Build history of the part. All positions in model axes, mm. Face numbers are marked on the shaded views. A direction names the side the tool comes from. Give positions to 0.01 mm unless a question says otherwise; leave off trailing zeros. Loops run counter-clockwise (first coordinate to the right, second up) from the corner with the lowest first, then second, coordinate; pieces in that order, holes last. Notation, with made-up numbers: (34.25, 16.5) -> (88.25, 16.5) arc R3 cw to (88.25, 20.5) -> close; hole circle Ø3 at (49, 49.5). An arc over 180 degrees is marked (long way). Answer in a Markdown table with one row per item. Add a question column.
from build123d import *

# Parameters (mm, degrees)
MAIN_BODY_DEPTH  = 77
LENS_CUT_DEPTH   = 3.1
END_RECESS_START = -77
END_RECESS_DEPTH = 1.05


with BuildPart() as part:
    # main_features_sketch → main_body (new, symmetric)
    with BuildSketch(Plane.XY):
        with BuildLine():
            ThreePointArc((24.721981093, -10.075200948), (21.063236898, -18.011630623), (12.946199947, -21.25))
            Line((12.946199947, -21.25), (-12.946199947, -21.25))
            ThreePointArc((-12.946199947, -21.25), (-21.063236898, -18.011630623), (-24.721981093, -10.075200948))
            Line((-24.721981093, -10.075200948), (-25.25, 0))
            Line((-25.25, 0), (-24.45, 0))
            Line((-24.45, 0), (-24.45, 0.6))
            Line((-24.45, 0.6), (-25.25, 0.6))
            Line((-25.25, 0.6), (-24.719878978, 10.11408323))
            ThreePointArc((-24.719878978, 10.11408323), (-21.049103134, 18.025020906), (-12.946199947, 21.25))
            Line((-12.946199947, 21.25), (12.946199947, 21.25))
            ThreePointArc((12.946199947, 21.25), (21.049103134, 18.025020906), (24.719878978, 10.11408323))
            Line((24.719878978, 10.11408323), (25.25, 0.6))
            Line((25.25, 0.6), (24.45, 0.6))
            Line((24.45, 0.6), (24.45, 0))
            Line((24.45, 0), (25.25, 0))
            Line((25.25, 0), (24.721981093, -10.075200948))
        make_face()
        with BuildLine():
            ThreePointArc((-23.124173837, -9.991463418), (-19.961869577, -16.85103163), (-12.946199947, -19.65))
            Line((-12.946199947, -19.65), (12.946199947, -19.65))
            ThreePointArc((12.946199947, -19.65), (19.961869577, -16.85103163), (23.124173837, -9.991463418))
            Line((23.124173837, -9.991463418), (23.5639518, -1.6))
            Line((23.5639518, -1.6), (22.85, -1.6))
            Line((22.85, -1.6), (22.85, 2.2))
            Line((22.85, 2.2), (23.558366806, 2.2))
            Line((23.558366806, 2.2), (23.12235695, 10.025069924))
            ThreePointArc((23.12235695, 10.025069924), (19.949653565, 16.86260504), (12.946199947, 19.65))
            Line((12.946199947, 19.65), (-12.946199947, 19.65))
            ThreePointArc((-12.946199947, 19.65), (-19.949653565, 16.86260504), (-23.12235695, 10.025069924))
            Line((-23.12235695, 10.025069924), (-23.558366806, 2.2))
            Line((-23.558366806, 2.2), (-22.85, 2.2))
            Line((-22.85, 2.2), (-22.85, -1.6))
            Line((-22.85, -1.6), (-23.5639518, -1.6))
            Line((-23.5639518, -1.6), (-23.124173837, -9.991463418))
        make_face(mode=Mode.SUBTRACT)
        with BuildLine():
            Line((-23.5639518, -1.6), (-23.124173837, -9.991463418))
            ThreePointArc((-23.124173837, -9.991463418), (-19.961869577, -16.85103163), (-12.946199947, -19.65))
            Line((-12.946199947, -19.65), (12.946199947, -19.65))
            ThreePointArc((12.946199947, -19.65), (19.961869577, -16.85103163), (23.124173837, -9.991463418))
            Line((23.124173837, -9.991463418), (23.5639518, -1.6))
            Line((23.5639518, -1.6), (22.85, -1.6))
            Line((22.85, -1.6), (22.85, 2.2))
            Line((22.85, 2.2), (23.558366806, 2.2))
            Line((23.558366806, 2.2), (23.12235695, 10.025069924))
            ThreePointArc((23.12235695, 10.025069924), (19.949653565, 16.86260504), (12.946199947, 19.65))
            Line((12.946199947, 19.65), (-12.946199947, 19.65))
            ThreePointArc((-12.946199947, 19.65), (-19.949653565, 16.86260504), (-23.12235695, 10.025069924))
            Line((-23.12235695, 10.025069924), (-23.558366806, 2.2))
            Line((-23.558366806, 2.2), (-22.85, 2.2))
            Line((-22.85, 2.2), (-22.85, -1.6))
            Line((-22.85, -1.6), (-23.5639518, -1.6))
        make_face()
    extrude(amount=MAIN_BODY_DEPTH, both=True)

    # lens_sketch → lens_cut (cut)
    with BuildSketch(Plane(origin=(0, 21.25, 0), x_dir=(1, 0, 0), z_dir=(0, 1, 0))):
        with BuildLine():
            Line((9.085700376, 58.2), (-9.085700376, 58.2))
            ThreePointArc((-9.085700376, 58.2), (-14.310724248, 56.035724248), (-16.475, 50.810700376))
            Line((-16.475, 50.810700376), (-16.475, 5.389299624))
            ThreePointArc((-16.475, 5.389299624), (-14.310724248, 0.164275752), (-9.085700376, -2))
            Line((-9.085700376, -2), (9.085700376, -2))
            ThreePointArc((9.085700376, -2), (14.310724248, 0.164275752), (16.475, 5.389299624))
            Line((16.475, 5.389299624), (16.475, 50.810700376))
            ThreePointArc((16.475, 50.810700376), (14.310724248, 56.035724248), (9.085700376, 58.2))
        make_face()
    extrude(amount=-LENS_CUT_DEPTH, mode=Mode.SUBTRACT)

    # Sketch1<3> → end_recess (cut)
    with BuildSketch(Plane.XY.offset(END_RECESS_START)):
        with BuildLine():
            Line((-23.5639518, -1.6), (-23.124173837, -9.991463418))
            ThreePointArc((-23.124173837, -9.991463418), (-19.961869577, -16.85103163), (-12.946199947, -19.65))
            Line((-12.946199947, -19.65), (12.946199947, -19.65))
            ThreePointArc((12.946199947, -19.65), (19.961869577, -16.85103163), (23.124173837, -9.991463418))
            Line((23.124173837, -9.991463418), (23.5639518, -1.6))
            Line((23.5639518, -1.6), (22.85, -1.6))
            Line((22.85, -1.6), (22.85, 2.2))
            Line((22.85, 2.2), (23.558366806, 2.2))
            Line((23.558366806, 2.2), (23.12235695, 10.025069924))
            ThreePointArc((23.12235695, 10.025069924), (19.949653565, 16.86260504), (12.946199947, 19.65))
            Line((12.946199947, 19.65), (-12.946199947, 19.65))
            ThreePointArc((-12.946199947, 19.65), (-19.949653565, 16.86260504), (-23.12235695, 10.025069924))
            Line((-23.12235695, 10.025069924), (-23.558366806, 2.2))
            Line((-23.558366806, 2.2), (-22.85, 2.2))
            Line((-22.85, 2.2), (-22.85, -1.6))
            Line((-22.85, -1.6), (-23.5639518, -1.6))
        make_face()
    end_recess = extrude(amount=END_RECESS_DEPTH, mode=Mode.SUBTRACT)

    # end_recess_2: end_recess across plane
    add(end_recess.mirror(Plane.XY), mode=Mode.SUBTRACT)


solid = part.part
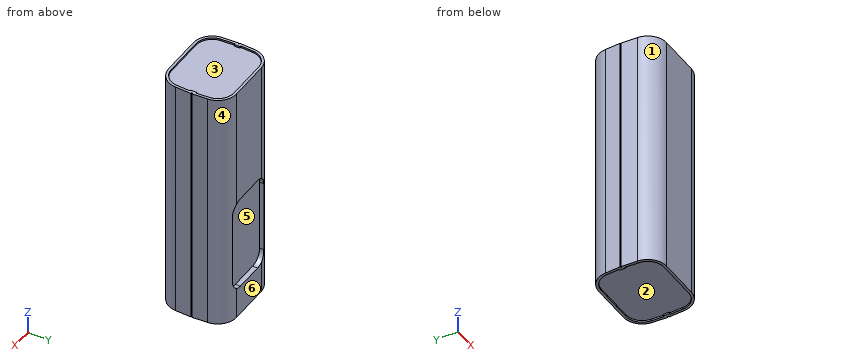
(1) 3-axis set-ups, long thin cutter, end or side, ignore diameter. For the marked faces 5 and 6: which of +Z, -Z, +X, -X, +Y, -Y reach the whole face in a straight line?
(2) Saw through at A-A, the plane z = -35. List the corners of the cut face in (x, y) (3 decimals).
(3) Flat gauge pins, fed straight in: pin 1 Ø4 at (y, z) = (13.5, -54) entering from -X; pin 2 Ø4 at (x, y) = (-17.5, 2.5) entering from +Z; pin 3 Ø12 at (x, y) = (7.5, -3.5) entering from -Z. Where does each tip first touch, or does it go through?
(4) Wall check: line 1 along Y through (x, z) = (3, -21.5); line 2 along Y through (x, z) = (13.5, 34); line 3 along Z through (x, y) = (-1.5, -8.5). Give the ranges that are in metal, low to high. Write a range as from..to.
(5) Saw through at D-D, the plane z = 66. List the corners of the cut face in (x, y).
(6) Two-plate mould, pull along Y, no slides. Class the marked faces 1, 2, 3 and 4: released by +Y, released by -Y, zero draft, split by the parting line, or undercut.
(7) Saw through at B-B, the plane x = -5. List the corners of the cut face in (y, z).
(8) Saw through at C-C, the plane y = -14.5. List the corners of the cut face in (x, z).
Worked answers:
| question | item | result |
|---|---|---|
| 1 | face 5 | +Y |
| 1 | face 6 | +Z, -Z, +X, -X, +Y |
| 2 | outline | (-25.25, 0) -> (-24.722, -10.075) arc R11.792 ccw to (-12.946, -21.25) -> (12.946, -21.25) arc R11.792 ccw to (24.722, -10.075) -> (25.25, 0) -> (24.45, 0) -> (24.45, 0.6) -> (25.25, 0.6) -> (24.72, 10.114) arc R11.792 ccw to (16.475, 20.71) -> (16.475, 18.15) -> (-16.475, 18.15) -> (-16.475, 20.71) arc R11.792 ccw to (-24.72, 10.114) -> (-25.25, 0.6) -> (-24.45, 0.6) -> (-24.45, 0) -> close |
| 3 | pin 1 | x = -24.56 |
| 3 | pin 2 | z = 75.95 |
| 3 | pin 3 | z = -75.95 |
| 4 | line 1 | -21.25..18.15 |
| 4 | line 2 | -21.24..21.24 |
| 4 | line 3 | -75.95..75.95 |
| 5 | outline | (-25.25, 0) -> (-24.72, -10.08) arc R11.79 ccw to (-12.95, -21.25) -> (12.95, -21.25) arc R11.79 ccw to (24.72, -10.08) -> (25.25, 0) -> (24.45, 0) -> (24.45, 0.6) -> (25.25, 0.6) -> (24.72, 10.11) arc R11.79 ccw to (12.95, 21.25) -> (-12.95, 21.25) arc R11.79 ccw to (-24.72, 10.11) -> (-25.25, 0.6) -> (-24.45, 0.6) -> (-24.45, 0) -> close |
| 6 | face 1 | released by -Y |
| 6 | face 2 | undercut |
| 6 | face 3 | undercut |
| 6 | face 4 | released by +Y |
| 7 | outline | (-21.25, -77) -> (-19.65, -77) -> (-19.65, -75.95) -> (19.65, -75.95) -> (19.65, -77) -> (21.25, -77) -> (21.25, -58.2) -> (18.15, -58.2) -> (18.15, 2) -> (21.25, 2) -> (21.25, 77) -> (19.65, 77) -> (19.65, 75.95) -> (-19.65, 75.95) -> (-19.65, 77) -> (-21.25, 77) -> close |
| 8 | outline | (-23.61, -77) -> (-21.8, -77) -> (-21.8, -75.95) -> (21.8, -75.95) -> (21.8, -77) -> (23.61, -77) -> (23.61, 77) -> (21.8, 77) -> (21.8, 75.95) -> (-21.8, 75.95) -> (-21.8, 77) -> (-23.61, 77) -> close |
